CAD build for the part. Positions are in the model's coordinates, mm. A direction names the side the tool comes from. Coordinates: 2 decimals unless noted, no trailing zeros. Loops run counter-clockwise (first coordinate to the right, second up) from the corner with the lowest first, then second, coordinate; pieces in that order, holes last. Notation, with made-up numbers: (-25, 87.25) -> (-5, 87.25) arc R11 ccw to (-5, 99.25) -> close; hole circle Ø4 at (-1.75, 39.5). An arc over 180 degrees is marked (long way). Write item = value, one per line. Start each with the question number.
(1) Tool access for faces 1 (the face through (-4, 14, 5)), 2 (the face through (0, 0, 0)): list every direction of +Z, -Z, +X, -X, +Y, -Y with a clear straight run to the whole face (end or side of a thin tool).
(2) Band-saw the part on C-C (y = -20). Write the cut outline in (x, z).
(3) Band-saw the part on B-B (x = -13). Write the cut outline in (y, z).
(4) Flat gauge pins, fed straight in: P1, Ø4.5, axis at x = 13, y = -20, coming from the +Z side; P2, Ø4.5, axis at x = 13, y = 20, coming from the -Z side; P3, Ø5, axis at y = 16.5, z = 6.5, coming from the -X side. Where does each tip first touch, or does it go through?
(5) Band-saw the part on D-D (z = 9). Write the cut outline in (x, y).
(6) Band-saw the part on A-A (y = 20). Write the cut outline in (x, z).
(7) Pull direction X, two halves, no side cores. Call faces 3 (the face through (-13.26, 18.017, 0.493)), 4 (the face through (4, 14, 5)), 5 (the face through (0.3, -25, 0.5)): +X half, -X half, draft (parallel to the pull), parting line (faces both ways), or undercut.
(8) Drill centre lines: line 1 (Y direction, x = 13, z = 0.35); line 2 (Z direction, x = 15, y = -2); line 3 (X direction, y = 8, z = 2.5). Where is each one in solid material? Low to high. Write a range as from..to.
Autodesk Inventor part; units mm, degrees
ref_plane "YZ Plane" through (0, 0, 0) normal (1, 0, 0) x (0, 1, 0)
ref_plane "XZ Plane" through (0, 0, 0) normal (0, 1, 0) x (-1, 0, 0)
ref_plane "XY Plane" through (0, 0, 0) normal (0, 0, 1) x (1, 0, 0)
sketch "Esboço1" plane through (0, 0, 0) normal (0, 0, 1) x (1, 0, 0)
  circle A0 centre (-13, -20) radius 2
  circle A1 centre (-13, 20) radius 2
  circle A2 centre (13, -20) radius 2
  circle A3 centre (13, 20) radius 2
  arc A4 (-15, 28) -> (-21, 22) centre (-15, 22) ccw
  line L0 (-21, 22) -> (-21, -38)
  arc A5 (-21, -38) -> (-15, -44) centre (-15, -38) ccw
  line L1 (-15, -44) -> (15, -44)
  arc A6 (15, -44) -> (21, -38) centre (15, -38) ccw
  line L2 (21, -38) -> (21, 22)
  arc A7 (21, 22) -> (15, 28) centre (15, 22) ccw
  line L3 (15, 28) -> (-15, 28)
  line L4 (-18, 25) -> (18, 25)
  line L5 (18, 25) -> (18, -25)
  line L6 (18, -25) -> (-18, -25)
  line L7 (-18, -25) -> (-18, 25)
  point P0 (0, 0)
extrude "Extrusão1" add sketch "Esboço1" along normal blind 1 contours L4 L5 L6 L7
sketch "Esboço2" plane through (0, 0, 1) normal (0, 0, 1) x (1, 0, 0)
  line L0 (-4, 24) -> (4, 24)
  line L1 (4, 24) -> (4, 14)
  line L2 (4, 14) -> (-4, 14)
  line L3 (-4, 14) -> (-4, 24)
  circle A0 centre (-13, 20) radius 2
  circle A1 centre (13, 20) radius 2
  line L4 (18, 25) -> (-18, 25)
  point P0 (0, 0)
  dimension "d7" = 8
  dimension "d8" = 10
  dimension "d10" = 7
  dimension "d12" = 1
revolve "Revolução1" add sketch "Esboço2" angle 180 about axis through (4, 14, 1) along (1, 0, 0) contours L0 L1 L2 L3
properties part number "Placa-Circuito"
Findings below:
q1.face_1 = +Z, -X, +Y, -Y
q1.face_2 = -Z, +X, -X, +Y, -Y
q2.outline = (-18, 0) -> (-15, 0) -> (-15, 1) -> (-18, 1) -> close; (-11, 0) -> (11, 0) -> (11, 1) -> (-11, 1) -> close; (15, 0) -> (18, 0) -> (18, 1) -> (15, 1) -> close
q3.outline = (-25, 0) -> (-22, 0) -> (-22, 1) -> (-25, 1) -> close; (-18, 0) -> (18, 0) -> (18, 1) -> (-18, 1) -> close; (22, 0) -> (25, 0) -> (25, 1) -> (22, 1) -> close
q4.P1 = 1
q4.P2 = 0
q4.P3 = -4
q5.outline = (-4, 8) -> (4, 8) -> (4, 20) -> (-4, 20) -> close
q6.outline = (-18, 0) -> (-15, 0) -> (-15, 1) -> (-18, 1) -> close; (-11, 0) -> (11, 0) -> (11, 1) -> (4, 1) -> (4, 9) -> (-4, 9) -> (-4, 1) -> (-11, 1) -> close; (15, 0) -> (18, 0) -> (18, 1) -> (15, 1) -> close
q7.face_3 = undercut
q7.face_4 = +X half
q7.face_5 = draft
q8.line_1 = -25..-22, -18..18, 22..25
q8.line_2 = 0..1
q8.line_3 = -4..4
